Part model, mm, in its own coordinate system. A direction names the side the tool comes from. Coordinates: 2 decimals unless noted, no trailing zeros. Write each loop counter-clockwise with the first axis right and the second up, starting at its lowest first coordinate (ties: lowest second). Pieces come first, ordered by that corner, then holes. Notation, with made-up numbers: (87.5, -16) - (99.5, -16) arc R32 cw to (99.5, 14) - close; hole circle Ø4 at (18.25, -24). An arc over 180 degrees is marked (long way). Write each question's results on one line, items separated by ' | '.
from build123d import *

# Parameters (mm, degrees)
BOSS_EXTRUDE1_DEPTH = 450
CUT_EXTRUDE1_DEPTH  = 449.5
SKETCH4_W           = 440
SKETCH4_H           = 340
CUT_EXTRUDE2_DEPTH  = 10
SKETCH7_R           = 0.125
BOSS_EXTRUDE2_DEPTH = 470


with BuildPart() as part:
    # Sketch2 → Boss-Extrude1 (new, symmetric)
    with BuildSketch(Plane(origin=(0, 0, 0), x_dir=(1, 0, 0), z_dir=(0, 1, 0))):
        with BuildLine():
            Line((-270, -200), (270, -200))
            ThreePointArc((270, -200), (291.213203436, -191.213203436), (300, -170))
            Line((300, -170), (300, 170))
            ThreePointArc((300, 170), (291.213203436, 191.213203436), (270, 200))
            Line((270, 200), (-270, 200))
            ThreePointArc((-270, 200), (-291.213203436, 191.213203436), (-300, 170))
            Line((-300, 170), (-300, -170))
            ThreePointArc((-300, -170), (-291.213203436, -191.213203436), (-270, -200))
        make_face()
    extrude(amount=BOSS_EXTRUDE1_DEPTH, both=True)

    # Sketch3 → Cut-Extrude1 (cut, symmetric)
    with BuildSketch(Plane(origin=(0, 0, 0), x_dir=(1, 0, 0), z_dir=(0, 1, 0))):
        with BuildLine():
            Line((-265, -200), (265, -200))
            Line((265, -200), (265, -192.5))
            ThreePointArc((265, -192.5), (284.445436483, -184.445436483), (292.5, -165))
            Line((292.5, -165), (300, -165))
            Line((300, -165), (300, 165))
            Line((300, 165), (292.5, 165))
            ThreePointArc((292.5, 165), (284.445436483, 184.445436483), (265, 192.5))
            Line((265, 192.5), (265, 200))
            Line((265, 200), (-265, 200))
            Line((-265, 200), (-265, 192.5))
            ThreePointArc((-265, 192.5), (-284.445436483, 184.445436483), (-292.5, 165))
            Line((-292.5, 165), (-300, 165))
            Line((-300, 165), (-300, -165))
            Line((-300, -165), (-292.5, -165))
            ThreePointArc((-292.5, -165), (-284.445436483, -184.445436483), (-265, -192.5))
            Line((-265, -192.5), (-265, -200))
        make_face()
    extrude(amount=CUT_EXTRUDE1_DEPTH, both=True, mode=Mode.SUBTRACT)

    # Sketch4 → Cut-Extrude2 (cut)
    with BuildSketch(Plane(origin=(0, 450, 0), x_dir=(1, 0, 0), z_dir=(0, 1, 0))):
        with Locations((50, 0)):
            Rectangle(SKETCH4_W, SKETCH4_H)
    extrude(amount=-CUT_EXTRUDE2_DEPTH, mode=Mode.SUBTRACT)

    # Sketch7 → Boss-Extrude2 (add)
    with BuildSketch(Plane(origin=(300, 0, 0), x_dir=(0, 0, -1), z_dir=(1, 0, 0))):
        with Locations((145, 449.75)):
            Circle(SKETCH7_R)
    extrude(amount=-BOSS_EXTRUDE2_DEPTH)


solid = part.part
(1) Flat gauge pins, fed straight in: P1, Ø2, axis at x = 295.5, y = 1, coming from the +Z side; P2, Ø6, axis at y = 88.5, z = -196.5, coming from the +X side; P3, Ø4, axis at y = 66.5, z = -198, coming from the -X side. Where does each tip first touch, or does it go through?
Return value:
P1: stops at z = 187.31 | P2: stops at x = 288.65 | P3: stops at x = -284.97
(2) Saw through at B-B on y = -314. Write the cut outline in (x, z).
Return value:
outline: (-300, -170) arc R30 ccw to (-270, -200) - (-265, -200) - (-265, -192.5) arc R27.5 cw to (-292.5, -165) - (-300, -165) - close; (-300, 165) - (-292.5, 165) arc R27.5 cw to (-265, 192.5) - (-265, 200) - (-270, 200) arc R30 ccw to (-300, 170) - close; (265, -200) - (270, -200) arc R30 ccw to (300, -170) - (300, -165) - (292.5, -165) arc R27.5 cw to (265, -192.5) - close; (265, 192.5) arc R27.5 cw to (292.5, 165) - (300, 165) - (300, 170) arc R30 ccw to (270, 200) - (265, 200) - close
(3) Saw through at D-D on x = -202.5. Write the cut outline in (y, z).
Return value:
outline: (-450, -200) - (-449.5, -200) - (-449.5, 200) - (-450, 200) - close; (449.5, -200) - (450, -200) - (450, 200) - (449.5, 200) - close
(4) 3-axis set-ups, long thin cutter, end or side, ignore diameter. For faces 4 (the cylindrical face through (-290.979, 6.3, -191.445)), 5 (the cylindrical face through (-284.66, 6.29, 184.23)): which of +Z, -Z, +X, -X, +Y, -Y reach the whole face in a straight line?
Return value:
face 4: -Z, -X, +Y, -Y | face 5: none
(5) Two-plate mould, pull along Y, no slides. Class faces 1 (the flat face through (-4, -450, -3)), 2 (the flat face through (-204, 449.5, -3)), 3 (the cylindrical face through (291.445, 6.3, -190.979)): released by +Y, released by -Y, zero draft, split by the parting line, or undercut.
Return value:
face 1: released by -Y | face 2: undercut | face 3: zero draft
(6) Wall check: line 1 (X direction, y = 286, z = 166.5); line 2 (Y direction, x = -197, z = 31); line 3 (Y direction, x = 51.5, z = 24). Give the ranges that are in metal, low to high. Write a range as from..to.
Return value:
line 1: x = -300..-292.46, 292.46..300 | line 2: y = -450..-449.5, 449.5..450 | line 3: y = -450..-449.5
(7) Saw through at C-C on z = -115. Write the cut outline in (x, y), then the cut area to 3 significant figures.
Return value:
outline: (-300, -450) - (300, -450) - (300, -449.5) - (-300, -449.5) - close; (-300, 449.5) - (-170, 449.5) - (-170, 450) - (-300, 450) - close; (270, 449.5) - (300, 449.5) - (300, 450) - (270, 450) - close | area: 380 mm^2
